Design review of the part built by this model. Coordinates are the model's own, in mm. Face numbers are marked on the shaded views. A direction names the side the tool comes from. Round coordinates to 2 decimals unless told otherwise and drop trailing zeros. Write each loop counter-clockwise with the first axis right and the second up, starting at its lowest first coordinate (ties: lowest second). Pieces come first, ordered by that corner, then holes. Notation, with made-up numbers: M -30,-38 L -18,-38 A22 ccw -18,-2 Z; hole C 43,-9.75 d1. An arc over 180 degrees is marked long. Use CSV: the item, a comma, the result in double quotes.
from build123d import *

# Parameters (mm, degrees)
CHAMFER_SIZE = 1


with BuildPart() as part:
    # AdditivePipe: sweep along a path in Sketch001
    with BuildLine(Plane.XY) as additivepipe_path:
        CenterArc((0, 0), 15, 0, 360)
    # Sketch → AdditivePipe (sweep)
    with BuildSketch(Plane.XZ):
        Polygon((1.75, 29), (1.75, 17), (11.75, 7), (11.75, 0), (13.75, 0), (13.75, 5), (15.25, 5), (15.25, 7), (13.75, 7), (3.75, 17), (3.75, 29), align=None)
    sweep(path=additivepipe_path.line)

    # Chamfer
    chamfer_edges = [part.edges().sort_by_distance(p)[0] for p in [
        (-3.75, 0, 29),
        (-13.75, 0, 0),
    ]]
    chamfer(chamfer_edges, length=CHAMFER_SIZE)


solid = part.part
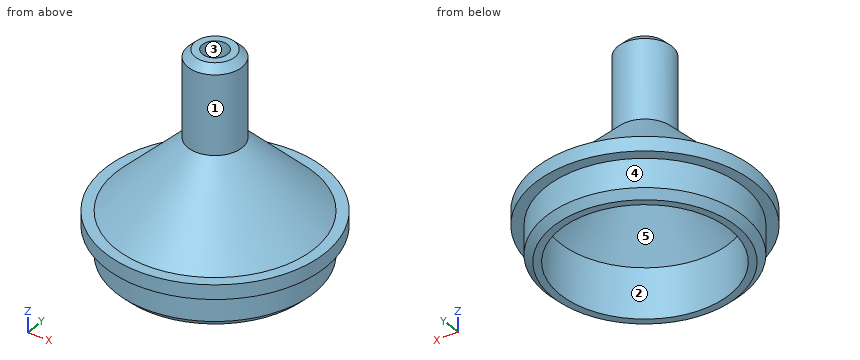
1) Machinability: for the marked faces 1 and 2, which of the approach directions +Z, -Z, +X, -X, +Y, -Y give a long, thin tool a straight path to every point of the face, cutting with its end or side? Answer none if there is none.
Answers:
face 1,"+Z"
face 2,"-Z"
2) Wall thickness on line 1 along Y through (x, z) = (0, 2.25); line 2 along Y through (x, z) = (0, 23); line 3 along X through (y, z) = (10, 7.5): over which ranges is each line inside the solid? List them lowest first. Write a range as [from, to].
Answers:
line 1,"[-13.75, -11.75], [11.75, 13.75]"
line 2,"[-3.75, -1.75], [1.75, 3.75]"
line 3,"[-8.69, -5.15], [5.15, 8.69]"
3) Add section A-A on z = 9.5. Write out the cut boundary in (x, y).
Answers:
outline,"C 0,0 d22.5; hole C 0,0 d18.5"
4) The part is to be moulded in two halves that separate along X. For the marked faces 3, 4 and 5, say which applies: released by +X, released by -X, zero draft, split by the parting line, or undercut.
Answers:
face 3,"undercut"
face 4,"split by the parting line"
face 5,"undercut"
5) For pin 1 Ø6 at (x, z) = (-3, 13.5) entering from -Y; pin 2 Ø1.5 at (x, y) = (11.5, -2.5) entering from +Z; pin 3 Ø2 at (x, y) = (0, 0) entering from -Z; pin 4 Ø8 at (x, z) = (-2.5, 20.5) entering from +Y, all flat-tipped, find the tip position at first contact; note any pin that passes through.
Answers:
pin 1,"y = -9.9"
pin 2,"z = 9.73"
pin 3,"through"
pin 4,"y = 3.85"
